from build123d import *

# Parameters (mm, degrees)
F1_ANGLE = 40
F2_DEPTH = 12.7
F3_DEPTH = 12.7


with BuildPart() as f1:
    # F0 (on Front) → F1 (revolve, symmetric)
    with BuildSketch(Plane.XZ) as f1_sk:
        Polygon((14.551543, -6.304409), (-5.839557, -6.304409), (-5.839557, -10.114409), (0, -10.114409), (0, -25.354409), (5.637471, -25.354409), (5.637471, -10.114409), (8.914071, -10.114409), (8.914071, -25.354409), (14.551543, -25.354409), (14.551543, -10.114409), align=None)
    revolve(axis=Axis((-35.485129, 0, -12.677205), (0, 0, 1)), revolution_arc=F1_ANGLE / 2)
    revolve(f1_sk.sketch, axis=Axis((-35.485129, 0, -12.677205), (0, 0, -1)), revolution_arc=F1_ANGLE / 2)

    # F0 (on Front) → F2 (join)
    with BuildSketch(Plane.XZ):
        Polygon((14.551543, 25.204011), (0, 0), (-3.299557, 1.905), (-5.839557, -2.494409), (-5.839557, -6.304409), (14.551543, -6.304409), (14.551543, 1.351308), (9.63061, 4.19241), (12.312471, 8.837529), (14.551543, 7.544801), align=None)
    extrude(amount=F2_DEPTH)

    # F0 (on Front) → F3 (join)
    with BuildSketch(Plane.XZ):
        Polygon((14.551543, 25.204011), (0, 0), (-3.299557, 1.905), (-5.839557, -2.494409), (-5.839557, -6.304409), (14.551543, -6.304409), (14.551543, 1.351308), (9.63061, 4.19241), (12.312471, 8.837529), (14.551543, 7.544801), align=None)
    extrude(amount=-F3_DEPTH)


solid = f1.part
Geometry: final body of the model. Coordinates: model frame, mm. A direction names the side the tool comes from. Round coordinates to 2 decimals unless told otherwise and drop trailing zeros. Loops run counter-clockwise (first coordinate to the right, second up) from the corner with the lowest first, then second, coordinate; pieces in that order, holes last.
Q1. Section D-D on z = 7. Return loops of the section in (x, y).
Q2. Section B-B on y = 7. Return loops of the section in (x, z) (3 decimals).
Q3. Material intervals for L1, parallel to Z at x = 12.25, y = 13.5; L2, parallel to X at y = 2, z = -6; L3, parallel to Y at x = -3.25, z = 0, sorted ascending.
Q4. Access query for faces 1 (the flat face through (14, -10, -6.304)), 2 (the flat face through (-1.63, -0.18, 0.94)), 3 (the flat face through (-5.84, 0, -4)). Directions: +Z, -Z, +X, -X, +Y, -Y. A direction counts if a zero-diameter tool reaches every point of the face in a straight line with its end or side. Return the directions, or none.
Q5. Pin query (flat end, axial travel): P1, Ø2.5, axis at x = -3, y = -2, coming from the -Z side; P2, Ø4, axis at x = 6.5, y = 4.5, coming from the +Z side; P3, Ø5, axis at x = -3.5, y = -3, coming from the +Z side (3 decimals); P4, Ø0.5, axis at x = -7, y = 6.5, coming from the +Z side. Return the tip coordinate at first contact, or that it passes through.
Q6. Section A-A on x = 10.5. Return loops of the section in (y, z).
Q7. Pull-direction query (Y, two-part tool) for faces 4 (the cylindrical face through (-5.84, 0.14, -8.24)), 5 (the cylindrical face through (5.637, 0.201, -17.628)), 6 (the flat face through (14.552, 0, 16)); classes: released by +Y, released by -Y, zero draft, split by the parting line, or undercut.
Q8. Section C-C on x = 1.75. Return loops of the section in (y, z).
Evaluation:
1. outline: (4.04, -12.7) - (11.25, -12.7) - (11.25, 12.7) - (4.04, 12.7) - close
2. outline: (-6.678, -10.114) - (-0.697, -10.114) - (-0.697, -25.354) - (5.037, -25.354) - (5.037, -10.114) - (8.359, -10.114) - (8.359, -25.354) - (14.059, -25.354) - (14.059, -6.304) - (14.552, -6.304) - (14.552, 1.351) - (9.631, 4.192) - (12.312, 8.838) - (14.552, 7.545) - (14.552, 25.204) - (0, 0) - (-3.3, 1.905) - (-5.84, -2.494) - (-5.84, -6.304) - (-6.678, -6.304) - close
3. L1: z = -25.35 to -6.3
3. L2: x = -5.84 to 14.55
3. L3: y = -12.7 to 12.7
4. face 1: -Z, +X, -Y
4. face 2: +Z, +Y, -Y
4. face 3: +Z, -X, +Y, -Y
5. P1: stops at z = -10.11
5. P2: stops at z = 14.72
5. P3: stops at z = 1.905
5. P4: passes through
6. outline: (-16.74, -25.35) - (16.74, -25.35) - (16.74, -6.3) - (12.7, -6.3) - (12.7, 3.69) - (-12.7, 3.69) - (-12.7, -6.3) - (-16.74, -6.3) - close; (-12.7, 5.7) - (12.7, 5.7) - (12.7, 18.19) - (-12.7, 18.19) - close
7. face 4: undercut
7. face 5: split by the parting line
7. face 6: zero draft
8. outline: (-13.55, -25.35) - (13.55, -25.35) - (13.55, -6.3) - (12.7, -6.3) - (12.7, 3.03) - (-12.7, 3.03) - (-12.7, -6.3) - (-13.55, -6.3) - close
